Design review of the part shown in the three views and the two pictorial views. Dimensions are in mm from the part's minimum x, y and z. A direction names the side the tool comes from. Round coordinates to 2 decimals unless told otherwise and drop trailing zeros. Loops run counter-clockwise (first coordinate to the right, second up) from the corner with the lowest first, then second, coordinate; pieces in that order, holes last. Notation, with made-up numbers: M -2,-16 L 11,-16 A20 ccw 11,-1 Z; hole C 31.25,77.5 d5. An arc over 180 degrees is marked long. Answer as CSV lines item,"result". Start each with the question number.
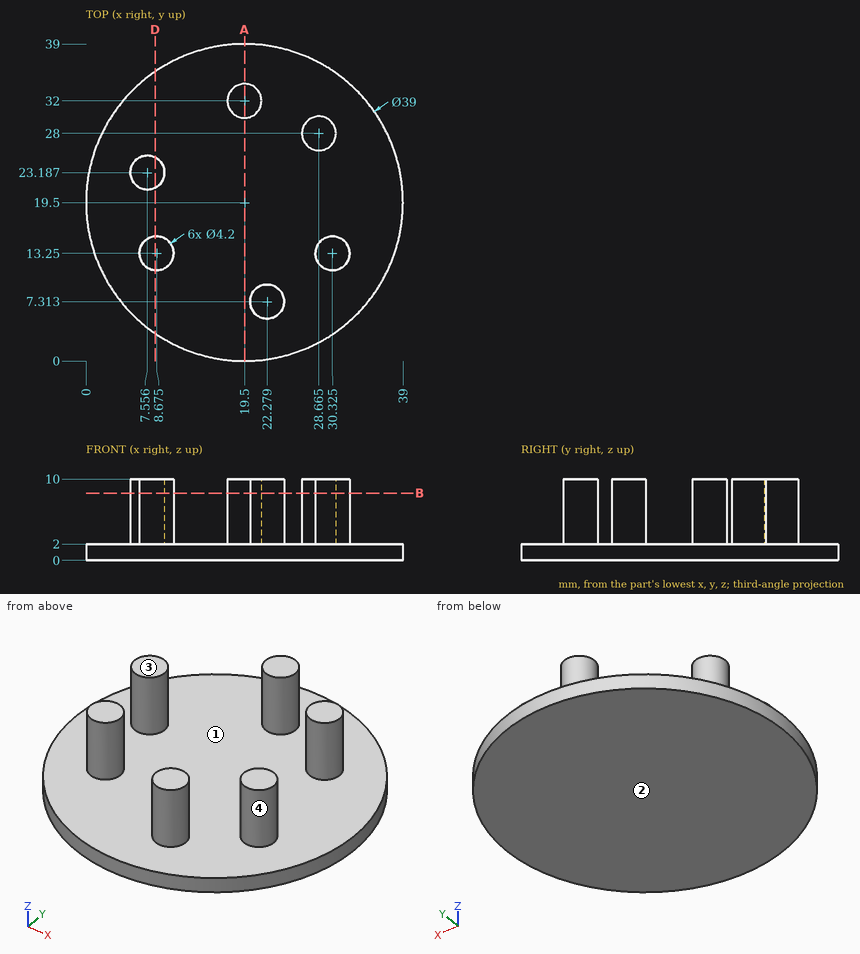
Item 1: Consider section D-D, the plane x = 8.5. Write out the cut boundary in (y, z).
Item 2: Insertion check: pin 1 Ø2 at (x, z) = (12, 7) entering from +Y; pin 2 Ø2 at (y, z) = (7.5, 2.5) entering from +X; pin 3 Ø8 at (x, y) = (9, 25.5) entering from -Z; pin 4 Ø4 at (x, z) = (30.5, 6.5) entering from +Y. Each pin has a flat end and moves straight along its axis. Give the tip position at first contact, or say it passes through.
Item 3: Tool access review of the marked faces 1 and 2: name each direction out of +Z, -Z, +X, -X, +Y, -Y from which nothing blocks a thin tool from reaching the whole face with its end or side.
Item 4: The part is to be moulded in two halves that separate along Y. For the marked faces 3 and 4, say which applies: +Y half, -Y half, draft (parallel to the pull), parting line (faces both ways), or undercut.
Item 5: To check wall thickness, follow line 1 (Z direction, x = 18, y = 15); line 2 (X direction, y = 33.5, z = 5.25); line 3 (Y direction, x = 31, z = 4). State the ranges of each line that lie inside material, in increasing order.
Item 6: Consider section B-B, the plane z = 8.25. Count the separate pieces of the cut face and the enclosed holes in it.
Item 7: Consider section A-A, the plane x = 19.5. Write out the cut boundary in (y, z), then the cut area to 3 significant figures.
Found:
1,outline,"M 3.4,0 L 35.6,0 L 35.6,2 L 25.06,2 L 25.06,10 L 21.31,10 L 21.31,2 L 15.34,2 L 15.34,10 L 11.16,10 L 11.16,2 L 3.4,2 Z"
2,pin 1,"passes through"
2,pin 2,"stops at x = 35.51"
2,pin 3,"stops at z = 0"
2,pin 4,"stops at y = 30.1"
3,face 1,"+Z"
3,face 2,"-Z, +X, -X, +Y, -Y"
4,face 3,"draft"
4,face 4,"undercut"
5,line 1,"z = 0 to 2"
5,line 2,"x = 18.03 to 20.97"
5,line 3,"y = 11.26 to 15.24"
6,separate pieces,"6"
6,enclosed holes,"0"
7,outline,"M 0,0 L 39,0 L 39,2 L 34.1,2 L 34.1,10 L 29.9,10 L 29.9,2 L 0,2 Z"
7,area,"112 mm^2"
